Check sheet for the modelled part. Datum: model origin and axes. Units: mm. A direction names the side the tool comes from. Give positions to 0.01 mm unless a question says otherwise; leave off trailing zeros. Order: outer loops, then holes, each group sorted by start corner. A loop starts at its lowest first (then second) coordinate and runs counter-clockwise, first axis right, second up.
Autodesk Inventor part; units mm, degrees
ref_plane "YZ Plane" through (0, 0, 0) normal (1, 0, 0) x (0, 1, 0)
ref_plane "XZ Plane" through (0, 0, 0) normal (0, 1, 0) x (-1, 0, 0)
ref_plane "XY Plane" through (0, 0, 0) normal (0, 0, 1) x (1, 0, 0)
sketch "Sketch1" plane through (0, 0, 0) normal (0, 0, 1) x (1, 0, 0)
  line L0 (381, -495.3) -> (-381, -495.3)
  line L1 (-381, -495.3) -> (-381, 495.3)
  line L2 (-381, 495.3) -> (381, 495.3)
  line L3 (381, 495.3) -> (381, -495.3)
  line L4 (381, -495.3) -> (-381, 495.3) construction
  line L5 (-381, -495.3) -> (381, 495.3) construction
  point P0 (0, 0)
  dimension "d0" = 762
  dimension "d1" = 990.6
extrude "Extrusion1" add sketch "Sketch1" along normal blind 25.4
sketch "Sketch2" plane through (0, 0, 25.4) normal (0, 0, 1) x (1, 0, 0)
  line L0 (-226.9738, 447.9746) -> (224.5353, 447.9746) construction
  line L1 (224.5353, 447.9746) -> (224.5353, -428.4841) construction
  line L2 (224.5353, -428.4841) -> (-226.9738, -428.4841) construction
  line L3 (-226.9738, -428.4841) -> (-226.9738, 447.9746) construction
  line L4 (175.8473, -419.5941) -> (175.8473, 245.0143)
  arc A0 (175.8473, 245.0143) -> (81.7255, 339.136) centre (81.7255, 245.0143) ccw
  line L5 (-226.9738, 0) -> (224.5353, 0)
  line L6 (81.7255, 339.136) -> (-0.7651, 339.136)
  line L7 (-1.2193, 447.9746) -> (-1.2193, -428.4841)
  line L8 (-0.7651, 339.136) -> (-109.9973, 339.136)
  line L9 (-197.5103, -325.9614) -> (-197.5103, 251.623)
  arc A1 (-109.9973, 339.136) -> (-197.5103, 251.623) centre (-109.9973, 251.623) ccw
  line L10 (175.8473, -419.5941) -> (-103.8776, -419.5941)
  arc A2 (-197.5103, -325.9614) -> (-103.8776, -419.5941) centre (-103.8776, -325.9614) ccw
  line L11 (60.5247, 66.1602) -> (15.8306, 66.1602)
  line L12 (15.8306, 66.1602) -> (15.8306, 127.3205)
  line L13 (15.8306, 127.3205) -> (124.6599, 127.3205)
  line L14 (124.6599, 127.3205) -> (124.6599, -305.458)
  line L15 (60.5247, 66.1602) -> (60.5247, -6.4131)
  line L16 (60.5247, -6.4131) -> (-76.9579, -6.4131)
  line L17 (-76.9579, -6.4131) -> (-76.9579, 229.6915)
  line L18 (-76.9579, 229.6915) -> (60.1228, 229.6915)
  line L19 (60.1228, 229.6915) -> (60.1228, 180.1667)
  line L20 (60.1228, 180.1667) -> (122.1436, 180.1667)
  line L21 (122.1436, 180.1667) -> (122.1436, 238.418)
  arc A3 (122.1436, 238.418) -> (69.7165, 290.8451) centre (69.7165, 238.418) ccw
  line L22 (69.7165, 290.8451) -> (-92.3667, 290.8451)
  arc A4 (-92.3667, 290.8451) -> (-141.7279, 241.4839) centre (-92.3667, 241.4839) ccw
  line L23 (-141.7279, 241.4839) -> (-141.7279, -27.6599)
  arc A5 (-141.7279, -27.6599) -> (-93.4193, -67.8148) centre (-89.1074, -13.4909) ccw
  line L24 (-93.4193, -67.8148) -> (58.494, -67.8148)
  line L25 (58.494, -67.8148) -> (58.494, -301.6299)
  line L26 (58.494, -301.6299) -> (-80.5428, -301.6299)
  line L27 (-80.5428, -301.6299) -> (-80.5428, -234.1224)
  line L28 (-80.5428, -234.1224) -> (-141.7279, -234.1224)
  line L29 (-141.7279, -234.1224) -> (-141.7279, -313.9932)
  arc A6 (-141.7279, -313.9932) -> (-93.2829, -362.4382) centre (-93.2829, -313.9932) ccw
  line L30 (-93.2829, -362.4382) -> (67.6797, -362.4382)
  arc A7 (67.6797, -362.4382) -> (124.6599, -305.458) centre (67.6797, -305.458) ccw
  line L31 (-141.7279, 241.4839) -> (-141.7279, 241.4839)
  line L32 (-381, 495.3) -> (-381, -495.3)
  line L33 (381, 495.3) -> (-381, 495.3)
  line L34 (381, -495.3) -> (381, 495.3)
  line L35 (-381, -495.3) -> (381, -495.3)
  point P0 (0, 0)
  point P1 (-1.2193, -67.8148)
  point P2 (-1.2193, -301.6299)
  dimension "d13" = 8.89
  dimension "d31" = 64.77
  dimension "d32" = 61.1536
extrude "Extrusion2" cut sketch "Sketch2" against normal up to surface (25.4 mm away) contours L14 A7 L30 L7 L26 L25 L24 L16 L15 L5 | L5 L15 L11 L12 L13 L14 | L30 A6 L29 L28 L27 L26 L7 | L7 L24 L25 L26 | L24 A5 L23 L5 L17 L16 L7 | L5 L23 A4 L22 L7 L18 L17 | L7 L22 A3 L21 L20 L19 L18 | L33 L34 L35 L32
(1) Set-up check for faces 1 (the face through (91, 180.167, 13)), 2 (the face through (-170.81, -391.44, 12.88)): record each of +Z, -Z, +X, -X, +Y, -Y from which the full face is reachable in a straight line by a thin tool's end or side.
Response values:
face 1: +Z, -Z
face 2: +Z, -Z, -X, -Y
(2) Cross-section at A-A on y = 40.5. Enter the section's corners in (x, z).
Response values:
outline: (-197.51, 0) - (-141.73, 0) - (-141.73, 25.4) - (-197.51, 25.4) - close; (-76.96, 0) - (60.52, 0) - (60.52, 25.4) - (-76.96, 25.4) - close; (124.66, 0) - (175.85, 0) - (175.85, 25.4) - (124.66, 25.4) - close
(3) Material ranges on L1, parallel to Y at x = -55.5, z = 16; L2, parallel to Y at x = 4.5, z = 6.25; L3, parallel to X at y = 224, z = 12.75, recorded low to high.
Response values:
L1: y = -419.59 to -362.44, -301.63 to -67.81, -6.41 to 229.69, 290.85 to 339.14
L2: y = -419.59 to -362.44, -6.41 to 229.69, 290.85 to 339.14
L3: x = -197.51 to -141.73, -76.96 to 60.12, 122.14 to 175.85
(4) Release check for a two-part mould opening along X. For faces 3 (the face through (-197.51, -41, 13)), 4 (the face through (-9, 229.692, 13)) record: released by +X, released by -X, zero draft, split by the parting line, or undercut.
Response values:
face 3: released by -X
face 4: undercut
(5) Cross-section at B-B on y = -153. Enter the section's corners in (x, z), then the cut area to 3 significant figures.
Response values:
outline: (-197.51, 0) - (-1.22, 0) - (-1.22, 25.4) - (-197.51, 25.4) - close; (124.66, 0) - (175.85, 0) - (175.85, 25.4) - (124.66, 25.4) - close
area: 6,290 mm2
(6) Cross-section at C-C on x = -124. Enter the section's corners in (y, z), then the cut area to 3 significant figures.
Response values:
outline: (-417.41, 0) - (-351.45, 0) - (-351.45, 25.4) - (-417.41, 25.4) - close; (-234.12, 0) - (-55.35, 0) - (-55.35, 25.4) - (-234.12, 25.4) - close; (279.38, 0) - (338.01, 0) - (338.01, 25.4) - (279.38, 25.4) - close
area: 7,710 mm2
